Can you work these out from the model? Positions are in its coordinate system, mm. A direction names the side the tool comes from. Round coordinates to 2 decimals unless told otherwise and drop trailing zeros. Write each loop counter-clockwise with the first axis right and the second up, starting at its lowest first coordinate (ties: lowest second). Pieces come first, ordered by that corner, then holes. Notation, with made-up numbers: M -33,68.25 L -29,68.25 A28 ccw -29,89.25 Z; hole C 53.5,-8 d6. An arc over 180 degrees is marked long. Answer in a Markdown table with one row per item. Add a question column.
(1) Suppose I cut it at C-C, the plane z = -94. Write out the boundary of the cut face in (x, y).
(2) Suppose I cut it at B-B, the plane x = -12.5. Write out the boundary of the cut face in (y, z).
(3) For faces 1 (the face through (-110, 4, -60)), 2 (the face through (-59, 115, -59)), which set-ups out of +Z, -Z, +X, -X, +Y, -Y let a thin tool reach every point of the face, with its end or its side?
(4) I'm going to push flat-ended pins straight in: pin 1 (2 mm diameter, centred on x = -115, z = -5, fed in from -Y); pin 2 (11 mm diameter, centred on x = -107, z = -12, fed in from -Y); pin 3 (0.5 mm diameter, centred on x = -105.5, z = -10, fed in from -Y). Where does each tip first touch, or does it pass through?
(5) If I drill on probe 1 along X at (y, z) = (99.5, -35.5); probe 2 along X at (y, z) = (5, -60), over which ranges is the centre line in solid material (lowest first)?
(6) Suppose I cut it at A-A, the plane y = 12. Write out the boundary of the cut face in (x, z).
Autodesk Inventor part; units mm, degrees
ref_plane "YZ Ebene" through (0, 0, 0) normal (1, 0, 0) x (0, 1, 0)
ref_plane "XZ Ebene" through (0, 0, 0) normal (0, 1, 0) x (-1, 0, 0)
ref_plane "XY Ebene" through (0, 0, 0) normal (0, 0, 1) x (1, 0, 0)
sketch "Sketch20" plane through (0, 0, 0) normal (0, 1, 0) x (-1, 0, 0)
  line L0 (0, 0) -> (120, 0)
  line L1 (120, 0) -> (120, -120)
  line L2 (120, -120) -> (0, -120)
  line L3 (0, -120) -> (0, 0)
  dimension "d58" = 120
  dimension "d59" = 120
extrude "Extrusion8" add sketch "Sketch20" along normal blind 115
sketch "Sketch21" plane through (0, 0, 0) normal (0, -1, 0) x (1, 0, 0)
  line L0 (-5, -5) -> (-115, -5)
  line L1 (-115, -5) -> (-115, -115)
  line L2 (-115, -115) -> (-5, -115)
  line L3 (-5, -115) -> (-5, -5)
  line L4 (0, -120) -> (0, 0)
  line L5 (0, 0) -> (-120, 0)
  dimension "d62" = 110
  dimension "d63" = 110
  dimension "d64" = 5
  dimension "d65" = 5
extrude "Extrusion9" cut sketch "Sketch21" against normal blind 110
sketch "Sketch22" plane through (0, 110, 0) normal (0, -1, 0) x (1, 0, 0)
  line L0 (-115, -115) -> (-115, -5)
  line L1 (-115, -5) -> (-5, -5)
  circle A0 centre (-105, -59) radius 5
  circle A1 centre (-105, -10) radius 5
  circle A2 centre (-47, -59) radius 5
  circle A3 centre (-47, -10) radius 5
  point P0 (0, 0)
  dimension "d68" = 10
  dimension "d69" = 5
  dimension "d70" = 49
  dimension "d71" = 58
  dimension "d72" = 10
  dimension "d73" = 10
  dimension "d74" = 10
  dimension "d75" = 10
extrude "Extrusion10" add sketch "Sketch22" along normal blind 5
sketch "Sketch23" plane through (-105, 105, -59) normal (0, -1, 0) x (1, 0, 0)
  circle A0 centre (0, 49) radius 5
  circle A1 centre (58, 0) radius 5
  circle A2 centre (58, 49) radius 5
  point P0 (105, 59)
  point P1 (0, 0)
  point P2 (0, 54)
  point P3 (58, 54)
hole "Hole2" at (-105, 105, -59) at (-105, 105, -10) at (-47, 105, -59) at (-47, 105, -10) direction (0, 1, 0) diameter 1.57 depth 5
fillet "Fillet5" radius 2 8 edges at (0, 57.5, 0) (-60, 115, 0) (0, 115, -60) (0, 57.5, -120) (-60, 115, -120) (-120, 115, -60) (-120, 57.5, -120) (-120, 57.5, 0)
sketch "Sketch24" plane through (0, 0, 0) normal (0, -1, 0) x (1, 0, 0)
  line L0 (-115, -5) -> (-105, -5)
  circle A0 centre (-115, -5) radius 5
  line L1 (-115, -5) -> (-5, -5)
  circle A1 centre (-5, -5) radius 5
  line L2 (-5, -5) -> (-5, -115)
  circle A2 centre (-5, -115) radius 5
  line L3 (-5, -115) -> (-115, -115)
  circle A3 centre (-115, -115) radius 5
  line L4 (-115, -115) -> (-115, -5)
  circle A4 centre (-115, -60) radius 5
  circle A5 centre (-5, -60) radius 5
  circle A6 centre (-60, -115) radius 5
  circle A7 centre (-60, -5) radius 5
  point P0 (0, 0)
  dimension "d86" = 10
  dimension "d87" = 10
  dimension "d88" = 10
  dimension "d89" = 10
  dimension "d90" = 10
  dimension "d91" = 10
  dimension "d92" = 10
  dimension "d93" = 10
extrude "Extrusion11" add sketch "Sketch24" against normal blind 10 contours L4 A0 L0 | L0 A0 L4 | A4 L4 | L4 A4 | A7 L1 | L1 A7 | L4 L3 A3 | A3 L3 L4 | A1 L2 L1 | L1 L2 A1 | A6 L3 | L3 A6 | A5 L2 | L2 A5 | L3 L2 A2 | A2 L2 L3
fillet "Fillet6" radius 2 8 edges at (-110, 10, -60) (-111.4645, 10, -111.4645) (-60, 10, -110) (-8.5355, 10, -111.4645) (-10, 10, -60) (-111.4645, 10, -8.5355) (-60, 10, -10) (-8.5355, 10, -8.5355)
sketch "Sketch25" plane through (0, 0, 0) normal (0, -1, 0) x (1, 0, 0)
  line L0 (-5, -8) -> (-5, -5)
  line L1 (-5, -63) -> (-5, -57)
  line L2 (-5, -115) -> (-115, -115)
  line L3 (-57, -5) -> (-63, -5)
  line L4 (-115, -57) -> (-115, -63)
  line L5 (-112, -5) -> (-115, -5)
  point P0 (0, 0)
  point P1 (-5, -60)
  point P2 (-60, -5)
  point P3 (-60, -115)
  point P4 (-115, -60)
hole "Hole3" at (-5, 0, -5) at (-5, 0, -60) at (-5, 0, -115) at (-60, 0, -5) at (-60, 0, -115) at (-115, 0, -60) at (-115, 0, -5) at (-115, 0, -115) direction (0, 1, 0) diameter 2.46 depth 8.8
properties part number "raspberry_box" material "S235JR"
Calculated:
| question | item | result |
|---|---|---|
| 1 | outline | M -120,0 L -115,0 L -115,110 L -5,110 L -5,0 L 0,0 L 0,113 A2 ccw -2,115 L -118,115 A2 ccw -120,113 Z |
| 2 | outline | M 0,-120 L 113,-120 A2 ccw 115,-118 L 115,-2 A2 ccw 113,0 L 0,0 L 0,-5 L 110,-5 L 110,-115 L 0,-115 Z |
| 3 | face 1 | -Y |
| 3 | face 2 | +Z, -Z, +X, -X, +Y |
| 4 | pin 1 | y = 8.8 |
| 4 | pin 2 | y = 105 |
| 4 | pin 3 | y = 110 |
| 5 | probe 1 | -120 to -115, -5 to 0 |
| 5 | probe 2 | -120 to -116.23, -113.77 to -110, -10 to -6.23, -3.77 to 0 |
| 6 | outline | M -120,-118 A2 ccw -118,-120 L -2,-120 A2 ccw 0,-118 L 0,-2 A2 ccw -2,0 L -118,0 A2 ccw -120,-2 Z; hole M -115,-115 L -5,-115 L -5,-5 L -115,-5 Z |
